Design review of the part built by this model. Coordinates are the model's own, in mm. Face numbers are marked on the shaded views. A direction names the side the tool comes from. Give positions to 0.01 mm unless a question says otherwise; leave off trailing zeros. Order: outer loops, then holes, each group sorted by start corner. A loop starts at its lowest first (then second) coordinate and runs counter-clockwise, first axis right, second up. Notation, with made-up numbers: (82.5, 42) -> (104.5, 42) arc R37 cw to (104.5, 81) -> close; hole circle Ø8 at (71.25, 67.5). An arc over 180 degrees is marked (long way). Return JSON: item names as keys, results as strings.
```python
from build123d import *

# Parameters (mm, degrees)
BOSS_EXTRUDE1_DEPTH = 40
FILLET3_R           = 7
FILLET4_R           = 7
FILLET5_R           = 7
SKETCH8_W           = 40
SKETCH8_H           = 119.824449513
BOSS_EXTRUDE2_DEPTH = 2
SKETCH9_W           = 40
SKETCH9_H           = 8
CUT_EXTRUDE6_DEPTH  = 5
FILLET6_R           = 3
FILLET7_R           = 3
SKETCH10_W          = 35
SKETCH10_H          = 100
CUT_EXTRUDE7_DEPTH  = 25
SKETCH11_R          = 5
CUT_EXTRUDE8_DEPTH  = 40
SKETCH12_W          = 36.007885592
SKETCH12_H          = 34
CUT_EXTRUDE9_DEPTH  = 3
CUT_EXTRUDE10_DEPTH = 4
SKETCH15_W          = 30.007885592
SKETCH15_H          = 8.507444754
CUT_EXTRUDE12_DEPTH = 4


with BuildPart() as part:
    # Sketch1 → Boss-Extrude1 (new body)
    with BuildSketch(Plane.XY):
        Polygon((-46.572492334, -83.741881942), (-67.776571631, 50.109646847), (-16.572492334, 50.109646847), (-16.572492334, -92.866074504), (-50.572492334, -92.866074504), (-50.572492334, -83.741881942), align=None)
    extrude(amount=BOSS_EXTRUDE1_DEPTH)

    # Fillet3
    fillet3_edges = [part.edges().sort_by_distance(p)[0] for p in [
        (-50.572492334, -92.866074504, 20),
    ]]
    fillet(fillet3_edges, radius=FILLET3_R)

    # Fillet4
    fillet4_edges = [part.edges().sort_by_distance(p)[0] for p in [
        (-16.572492334, 50.109646847, 20),
    ]]
    fillet(fillet4_edges, radius=FILLET4_R)

    # Fillet5
    fillet5_edges = [part.edges().sort_by_distance(p)[0] for p in [
        (-67.776571631, 50.109646847, 20),
    ]]
    fillet(fillet5_edges, radius=FILLET5_R)

    # Sketch8 → Boss-Extrude2 (add)
    with BuildSketch(Plane(origin=(-58.373554794, -9.247242044, 0), x_dir=(0, 0, 1), z_dir=(-0.987683688709488, -0.15646383306444783, 0))):
        with Locations((20, -15.511355434)):
            Rectangle(SKETCH8_W, SKETCH8_H)
    extrude(amount=BOSS_EXTRUDE2_DEPTH)

    # Sketch9 → Cut-Extrude6 (cut)
    with BuildSketch(Plane(origin=(-60.348922171, -9.56016971, 0), x_dir=(0, 0, 1), z_dir=(-0.987683688709488, -0.1564638330644479, 0))):
        with Locations((20, -71.106750349)):
            Rectangle(SKETCH9_W, SKETCH9_H)
    extrude(amount=-CUT_EXTRUDE6_DEPTH, mode=Mode.SUBTRACT)

    # Fillet6
    # the kernel refuses this fillet: 3 mm, written as the material it takes off along each edge
    with BuildSketch(Plane(origin=(-50.572492334, -83.741881942, -8.262362342), x_dir=(1, 0, 0), z_dir=(0, 0, 1))) as fillet6_piece_1:
        with BuildLine():
            CenterArc((3.057167778, -2.798042747), FILLET6_R, 111.143346589, 78.555093673)
            Line((0.100043612, -3.303430385), (-0.195668805, -3.353969149))
            ThreePointArc((-0.195668805, -3.353969149), (-0.3, -2.124192562), (-0.3, 0))
            Line((-0.3, 0), (0, 0.3))
            ThreePointArc((0, 0.3), (0.987530106, 0.3), (1.866849455, 0.279804275))
            Line((1.866849455, 0.279804275), (1.975060211, 0))
        make_face()
    extrude(amount=56.524724683, mode=Mode.SUBTRACT)
    with BuildSketch(Plane(origin=(-49.849142787, -75.840412432, -7.5), x_dir=(-0.15646383306444783, 0.9876836887094879, 0), z_dir=(0, 0, 1))) as fillet6_piece_2:
        with BuildLine():
            CenterArc((FILLET6_R, -FILLET6_R), FILLET6_R, 90, 90)
            Line((0, -FILLET6_R), (-FILLET6_R * 0.02, -FILLET6_R))
            Line((-FILLET6_R * 0.02, -FILLET6_R), (-FILLET6_R * 0.02, FILLET6_R * 0.02))
            Line((-FILLET6_R * 0.02, FILLET6_R * 0.02), (FILLET6_R, FILLET6_R * 0.02))
            Line((FILLET6_R, FILLET6_R * 0.02), (FILLET6_R, 0))
        make_face()
    extrude(amount=55, mode=Mode.SUBTRACT)

    # Fillet7
    fillet7_edges = [part.edges().sort_by_distance(p)[0] for p in [
        (-44.284869011, -79.008828021, 0),
        (-44.284869011, -79.008828021, 40),
        (-46.128222901, -83.350722359, 0),
        (-46.128222901, -83.350722359, 40),
    ]]
    fillet(fillet7_edges, radius=FILLET7_R)

    # Sketch10 → Cut-Extrude7 (cut)
    with BuildSketch(Plane(origin=(-16.572492334, 0, 0), x_dir=(0, 0, -1), z_dir=(1, 0, 0))):
        with Locations((-20, -37.866074504)):
            Rectangle(SKETCH10_W, SKETCH10_H)
    extrude(amount=-CUT_EXTRUDE7_DEPTH, mode=Mode.SUBTRACT)

    # Sketch11 → Cut-Extrude8 (cut)
    with BuildSketch(Plane.XZ.offset(-12.133925496)):
        with Locations(Location((-24.692244137, 10, 0), (0, 0, 270))):
            Circle(SKETCH11_R)
    extrude(amount=-CUT_EXTRUDE8_DEPTH, mode=Mode.SUBTRACT)

    # Sketch12 → Cut-Extrude9 (cut)
    with BuildSketch(Plane(origin=(0, 50.109646847, 0), x_dir=(1, 0, 0), z_dir=(0, 1, 0))):
        with Locations((-41.57643513, -20)):
            Rectangle(SKETCH12_W, SKETCH12_H)
    extrude(amount=-CUT_EXTRUDE9_DEPTH, mode=Mode.SUBTRACT)

    # Sketch14 → Cut-Extrude10 (cut)
    with BuildSketch(Plane(origin=(0, 47.109646847, 0), x_dir=(1, 0, 0), z_dir=(0, 1, 0))):
        with BuildLine():
            Line((-48.580377926, -23.212665104), (-48.580377926, -9))
            Line((-48.580377926, -9), (-53.580377926, -9))
            Line((-53.580377926, -9), (-53.580377926, -23.334974507))
            ThreePointArc((-53.580377926, -23.334974507), (-50.787463759, -35.24813089), (-48.580377926, -23.212665104))
        make_face()
        with BuildLine():
            Line((-35.273431744, -9.008916267), (-30.273436234, -9.015616726))
            Line((-30.273436234, -9.015616726), (-30.292646413, -23.350578361))
            ThreePointArc((-30.292646413, -23.350578361), (-33.101522793, -35.259981286), (-35.292478017, -23.22156861))
            Line((-35.292478017, -23.22156861), (-35.273431744, -9.008916267))
        make_face()
    extrude(amount=-CUT_EXTRUDE10_DEPTH, mode=Mode.SUBTRACT)

    # Sketch15 → Cut-Extrude12 (cut)
    with BuildSketch(Plane(origin=(0, 47.109646847, 0), x_dir=(1, 0, 0), z_dir=(0, 1, 0))):
        with Locations((-38.57643513, -7.253722377)):
            Rectangle(SKETCH15_W, SKETCH15_H)
    extrude(amount=-CUT_EXTRUDE12_DEPTH, mode=Mode.SUBTRACT)


solid = part.part
```
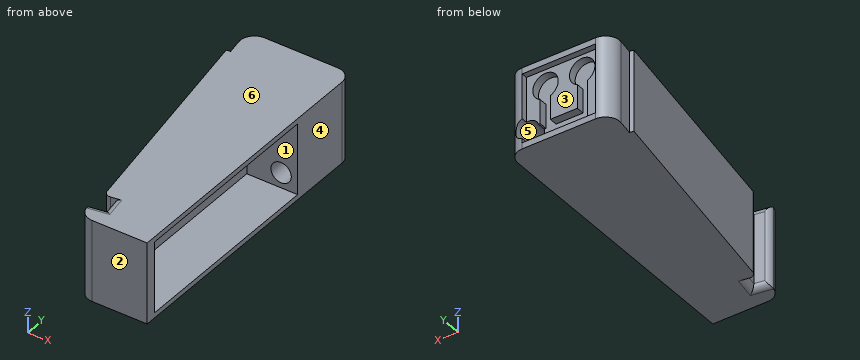
Item 1: Machinability: for the marked faces 1, 2 and 3, which of the approach directions +Z, -Z, +X, -X, +Y, -Y give a long, thin tool a straight path to every point of the face, cutting with its end or side? Answer none if there is none.
Result set:
{"face 1": "+X", "face 2": "+Z, -Z, +X, -X, -Y", "face 3": "+Y"}
Item 2: Add section C-C (z = 29). Give the boundary of the cut face in (x, y).
Result set:
{"outline": "(-67.3, 34.29) -> (-50.32, -72.88) arc R3 ccw to (-46.89, -75.37) -> (-44.91, -75.06) -> (-43.66, -82.96) -> (-48.6, -83.74) arc R3 ccw to (-50.47, -87.05) arc R7 ccw to (-43.57, -92.87) -> (-16.57, -92.87) -> (-16.57, -87.87) -> (-41.57, -87.87) -> (-41.57, 12.13) -> (-16.57, 12.13) -> (-16.57, 43.11) arc R7 ccw to (-23.57, 50.11) -> (-23.57, 47.11) -> (-26.69, 47.11) -> (-26.69, 43.11) -> (-39.19, 43.11) -> (-39.19, 47.11) -> (-44.69, 47.11) -> (-44.69, 43.11) -> (-57.19, 43.11) -> (-57.19, 47.11) -> (-59.58, 47.11) -> (-59.58, 50.11) arc R7 ccw to (-66.49, 42.01) -> (-65.32, 34.61) -> close"}
Item 3: Add section D-D (y = 30). Give the boundary of the cut face in (x, z), plus the area to 3 significant figures.
Result set:
{"outline": "(-66.62, 0) -> (-16.57, 0) -> (-16.57, 40) -> (-66.62, 40) -> close; hole circle Ø10 at (-24.69, 10)", "area": "1,920 mm^2"}
Item 4: Mouldability with a two-part tool opening along Z and no side actions: class the marked faces 4, 5 and 6 as released by +Z, released by -Z, zero draft, split by the parting line, or undercut.
Result set:
{"face 4": "zero draft", "face 5": "undercut", "face 6": "released by +Z"}
Item 5: Add section B-B (y = -4). Give the boundary of the cut face in (x, z).
Result set:
{"outline": "(-61.23, 0) -> (-16.57, 0) -> (-16.57, 2.5) -> (-41.57, 2.5) -> (-41.57, 37.5) -> (-16.57, 37.5) -> (-16.57, 40) -> (-61.23, 40) -> close"}
Item 6: Wall thickness on L1, parallel to Y at x = -28, z = 18; L2, parallel to Z at x = -33.5, y = -83.5; L3, parallel to Y at x = -35.5, z = 29.5: over which ranges is each line inside the solid? List them lowest first. Write a range as [from, to].
Result set:
{"L1": "y = [-92.87, -87.87], [12.13, 47.11]", "L2": "z = [0, 2.5], [37.5, 40]", "L3": "y = [-92.87, -87.87], [12.13, 43.11]"}
Item 7: Add section A-A (z = 8). Give the boundary of the cut face in (x, y).
Result set:
{"outline": "(-67.3, 34.29) -> (-50.32, -72.88) arc R3 ccw to (-46.89, -75.37) -> (-44.91, -75.06) -> (-43.66, -82.96) -> (-48.6, -83.74) arc R3 ccw to (-50.47, -87.05) arc R7 ccw to (-43.57, -92.87) -> (-16.57, -92.87) -> (-16.57, -87.87) -> (-41.57, -87.87) -> (-41.57, 12.13) -> (-29.27, 12.13) -> (-29.27, 43.11) -> (-53.58, 43.11) -> (-53.58, 47.11) -> (-59.58, 47.11) -> (-59.58, 50.11) arc R7 ccw to (-66.49, 42.01) -> (-65.32, 34.61) -> close; (-20.11, 12.13) -> (-16.57, 12.13) -> (-16.57, 43.11) arc R7 ccw to (-20.11, 49.19) -> close"}
Item 8: For pin 1 (2.5 mm diameter, centred on y = 45.5, z = 3.5, fed in from -X); pin 2 (2 mm diameter, centred on y = -41, z = 12, fed in from -X); pin 3 (10 mm diameter, centred on y = -35.5, z = 21.5, fed in from -X), all flat-tipped, find the tip position at first contact; note any pin that passes through.
Result set:
{"pin 1": "stops at x = -66.49", "pin 2": "stops at x = -55.53", "pin 3": "stops at x = -57.03"}
